The drawing under review shows one solid part. Ordinate dimensions are in mm from its lowest x, y, z. Give positions to 0.01 mm unless a question says otherwise; leave off trailing zeros. Write each loop counter-clockwise with the first axis right and the second up, starting at its lowest first coordinate (ties: lowest second). Pieces come first, ordered by that corner, then holes. Notation, with made-up numbers: M -15,-29.75 L 13,-29.75 A24 cw 13,0.25 Z; hole C -26.75,-2 d6. An arc over 180 degrees is marked long. Answer as a JSON object with one key per item and string values. Group by question number.
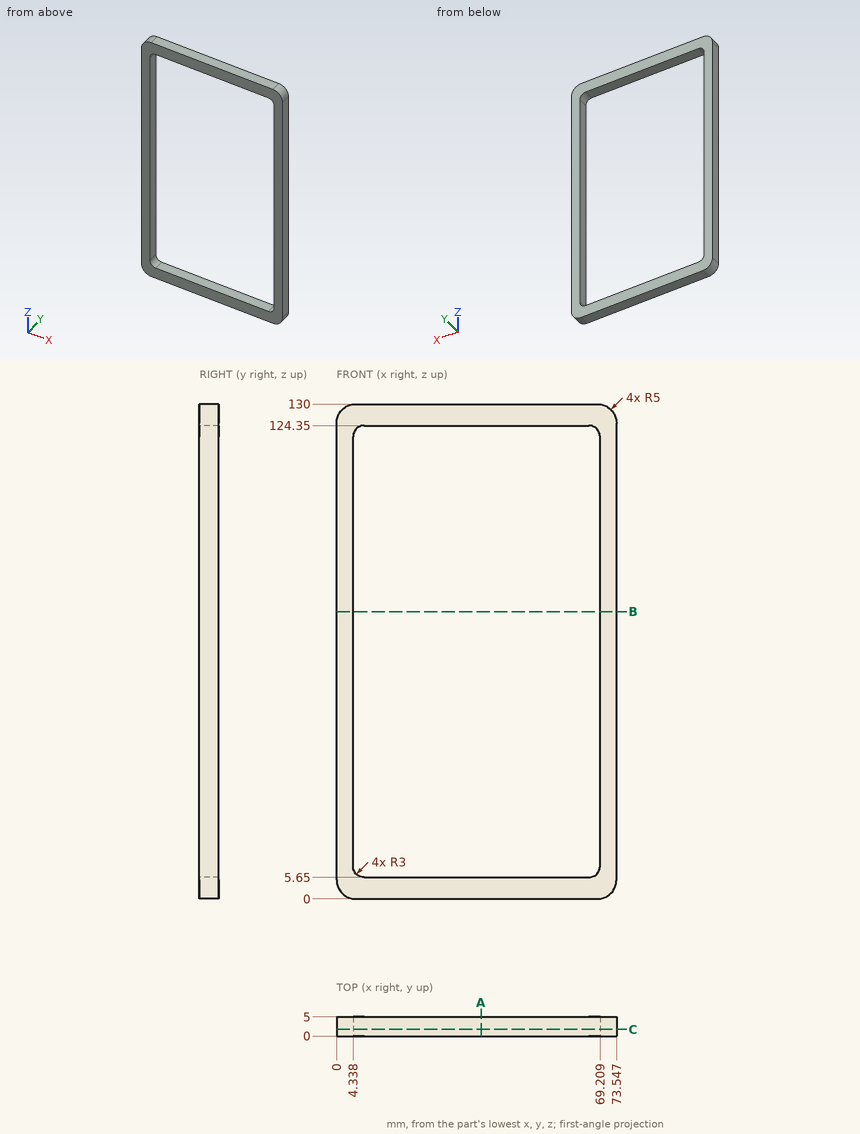
Item 1: To check wall thickness, follow probe 1 along X at (y, z) = (0.4, 118.5); probe 2 along Z at (x, y) = (55.5, 3.6). State the ranges of each line that lie inside material, in increasing order.
Item 2: Consider section B-B (z = 75.5). Give the boundary of the cut face in (x, y).
Item 3: Insertion check: P1, Ø1.5, axis at x = 47.5, y = 3.5, coming from the -Z side. The pin has a flat end and moves straight along its axis. Give the tip position at first contact, or say it passes through.
Item 4: Consider section A-A (x = 38). Give the boundary of the cut face in (y, z).
Item 5: Consider section C-C (y = 1.75). Give the boundary of the cut face in (x, z), plus the area to 3 significant figures.
Result set:
{
 "1": {"probe 1": "x = 0 to 4.34, 69.21 to 73.55", "probe 2": "z = 0 to 5.65, 124.35 to 130"},
 "2": {"outline": "M 0,0 L 4.34,0 L 4.34,5 L 0,5 Z; M 69.21,0 L 73.55,0 L 73.55,5 L 69.21,5 Z"},
 "3": {"P1": "stops at z = 0"},
 "4": {"outline": "M 0,0 L 5,0 L 5,5.65 L 0,5.65 Z; M 0,124.35 L 5,124.35 L 5,130 L 0,130 Z"},
 "5": {"outline": "M 0,5 A5 ccw 5,0 L 68.55,0 A5 ccw 73.55,5 L 73.55,125 A5 ccw 68.55,130 L 5,130 A5 ccw 0,125 Z; hole M 4.34,8.65 A3 ccw 7.34,5.65 L 66.21,5.65 A3 ccw 69.21,8.65 L 69.21,121.35 A3 ccw 66.21,124.35 L 7.34,124.35 A3 ccw 4.34,121.35 Z", "area": "1,850 mm^2"}
}
